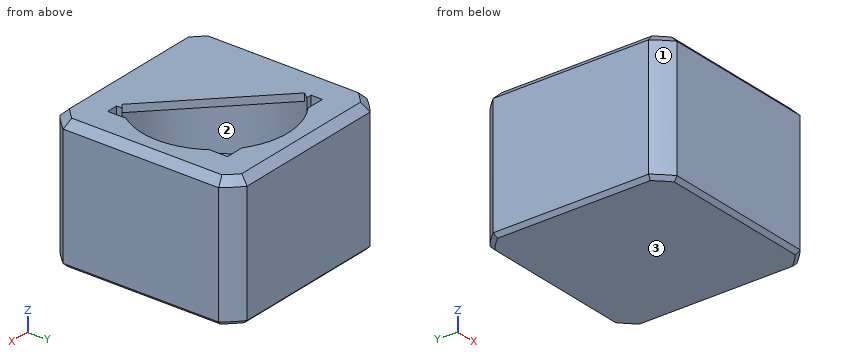
```python
from build123d import *

# Parameters (mm, degrees)
SKETCH_R        = 32.5
PAD_DEPTH       = 35
POCKET_DEPTH    = 22
SKETCH002_R     = 19.5
POCKET001_DEPTH = 22
POCKET002_DEPTH = 35.001
PAD001_DEPTH    = 2
CHAMFER_SIZE    = 2
CHAMFER001_SIZE = 1


with BuildPart() as part:
    # Sketch → Pad (new body)
    with BuildSketch(Plane.XY):
        Circle(SKETCH_R)
    extrude(amount=PAD_DEPTH)

    # Sketch001 (on Face3 of Pad) → Pocket (cut)
    with BuildSketch(Plane.XY.offset(35)):
        Polygon((-16, 16), (16, 16), (16, -16), (13, -16), (13, 13), (-16, 13), align=None)
    extrude(amount=-POCKET_DEPTH, mode=Mode.SUBTRACT)

    # Sketch002 (on Face3 of Pocket) → Pocket001 (cut)
    with BuildSketch(Plane.XY.offset(35)):
        Circle(SKETCH002_R)
    extrude(amount=-POCKET001_DEPTH, mode=Mode.SUBTRACT)

    # Sketch003 (on Face3 of Pocket001) → Pocket002 (cut, through all)
    with BuildSketch(Plane.XY.offset(35)):
        Polygon((25, 25), (25, -25), (67.494446, -25), (72.347168, 49.819519), (-56.328224, 49.819519), (-56.328224, -44.339888), (22.106388, -44.339888), (28.22, -25), (-25, -25), (-25, 25), align=None)
    extrude(amount=-POCKET002_DEPTH, mode=Mode.SUBTRACT)

    # Sketch004 (on Face4 of Pocket002) → Pad001 (join)
    with BuildSketch(Plane.XY.offset(35)):
        with BuildLine():
            ThreePointArc((-17.789269, 13.103439), (-15.397541, -15.845313), (13.607864, -17.406443))
            Line((-17.789269, 13.103439), (13.607864, -17.406443))
        make_face()
    extrude(amount=-PAD001_DEPTH)

    # Chamfer
    chamfer_edges = [part.edges().sort_by_distance(p)[0] for p in [
        (0, -25, 35),
        (22.98097, -22.98097, 35),
        (25, 0, 35),
        (22.98097, 22.98097, 35),
        (0, 25, 35),
        (-22.98097, 22.98097, 35),
        (-25, 0, 35),
        (-22.98097, -22.98097, 35),
    ]]
    chamfer(chamfer_edges, length=CHAMFER_SIZE)

    # Chamfer001
    chamfer001_edges = [part.edges().sort_by_distance(p)[0] for p in [
        (25, 0, 0),
        (22.98097, -22.98097, 0),
        (0, -25, 0),
        (-22.98097, -22.98097, 0),
        (-25, 0, 0),
        (-22.98097, 22.98097, 0),
        (0, 25, 0),
        (22.98097, 22.98097, 0),
    ]]
    chamfer(chamfer001_edges, length=CHAMFER001_SIZE)


solid = part.part
```
Check sheet for the modelled part. Datum: model origin and axes. Units: mm. Face numbers are marked on the shaded views. Round coordinates to 2 decimals unless told otherwise and drop trailing zeros. Write each loop counter-clockwise with the first axis right and the second up, starting at its lowest first coordinate (ties: lowest second). Pieces come first, ordered by that corner, then holes. Notation, with made-up numbers: M 50.25,29.25 L 60.25,29.25 A7 ccw 60.25,38.25 Z; hole C 11,73.25 d9. An arc over 180 degrees is marked long. Write item = value, one per line. Start each with the question number.
1. Scan lines: line 1 (X direction, y = 14, z = 25); line 2 (Y direction, x = -15.5, z = 30); line 3 (X direction, y = 0, z = 19). Record each from-to range of solid material in increasing order. Write a range as [from, to].
2. Section check B-B, the plane x = 9.5. Record the cut outline in (y, z), then the cut area to 3 significant figures.
3. Section check A-A, the plane z = 15. Record the cut outline in (x, y).
4. Section check C-C, the plane y = 2. Record the cut outline in (x, z), then the cut area to 3 significant figures.
5. Release check for a two-part mould opening along X. For the marked faces 1, 2 and 3 record: pulls with the +X half, pulls with the -X half, needs draft (parallel to the pull), parting line crosses it, or undercut.
6. Section check D-D, the plane x = -18.5. Record the cut outline in (y, z).
Results found:
q1.line_1 = [-25, -16], [16, 25]
q1.line_2 = [-25, -11.83], [11.83, 13], [16, 25]
q1.line_3 = [-25, -19.5], [19.5, 25]
q2.outline = M -25,1 L -24,0 L 24,0 L 25,1 L 25,33 L 23,35 L 17.03,35 L 17.03,13 L -17.03,13 L -17.03,33 L -13.41,33 L -13.41,35 L -23,35 L -25,33 Z
q2.area = 1,000 mm^2
q3.outline = M -25,-20.77 A32.5 ccw -20.77,-25 L 20.77,-25 A32.5 ccw 25,-20.77 L 25,20.77 A32.5 ccw 20.77,25 L -20.77,25 A32.5 ccw -25,20.77 Z; hole M -16,13 L -14.53,13 A19.5 ccw 13,-14.53 L 13,-16 L 16,-16 L 16,-11.15 A19.5 ccw 16,11.15 L 16,16 L 11.15,16 A19.5 ccw -11.15,16 L -16,16 Z
q4.outline = M -25,1 L -24,0 L 24,0 L 25,1 L 25,33 L 23,35 L 19.4,35 L 19.4,13 L -19.4,13 L -19.4,33 L -6.36,33 L -6.36,35 L -23,35 L -25,33 Z
q4.area = 918 mm^2
q5.face_1 = pulls with the -X half
q5.face_2 = undercut
q5.face_3 = needs draft
q6.outline = M -25,1 L -24,0 L 24,0 L 25,1 L 25,33 L 23,35 L -23,35 L -25,33 Z; hole M -6.16,13 L 6.16,13 L 6.16,33 L -6.16,33 Z
